Geometry check sheet. Reference: the model listing, model coordinates, mm. A direction names the side the tool comes from. Round coordinates to 2 decimals unless told otherwise and drop trailing zeros. Order: outer loops, then holes, each group sorted by start corner. A loop starts at its lowest first (then second) coordinate and runs counter-clockwise, first axis right, second up. Notation, with made-up numbers: (19.25, -22) - (76.25, -22) arc R25 cw to (76.25, -2) - close; hole circle Ø3 at (61.25, -19). An arc over 180 degrees is marked (long way). Return JSON: item names as keys, results as strings. Group by question number.
Q1. Draft check along Z on faces 1 (the flat face through (15, 11.847, 54)), 2 (the flat face through (-11, 36, 46.917)), 3 (the flat face through (-12, 22, 71.097)). Enter one of: pulls with the +Z half, pulls with the -Z half, needs draft (parallel to the pull), parting line crosses it, or undercut.
Q2. Sectioned sample at B-B, the plane y = 31.5. Record the cut outline in (x, z).
Q3. Sectioned sample at C-C, the plane y = 25.5. Record the cut outline in (x, z).
Q4. Tool access check on faces 4 (the flat face through (1, 22, 33.5)), 5 (the flat face through (-12, 22, 38.398)), 6 (the flat face through (4, 39.2, 93)), 7 (the flat face through (16.876, 37, 54)), 8 (the flat face through (1, 22, 58)). Record the directions out of +Z, -Z, +X, -X, +Y, -Y that give a thin tool (end or side, any length) a straight path to the whole face; none if there is none.
Q5. Gauge pin test, flat ends, axial feed: pin 1 Ø0.8 at (x, z) = (-12, 39.5) entering from -Y; pin 2 Ø3 at (y, z) = (2, 9) entering from -X; pin 3 Ø2.5 at (x, y) = (-10, 7.5) entering from -Z. Record the tip position at first contact, or that the pin passes through.
Q6. Material ranges on line 1 along Y through (x, z) = (12, 81.5); line 2 along Y through (x, z) = (5.5, 32); line 3 along Y through (x, z) = (-9.75, 55), recorded low to high.
Q7. Sectioned sample at D-D, the plane x = -8. Record the cut outline in (y, z).
```python
from build123d import *

# Parameters (mm, degrees)
BOSS_EXTRUDE1_DEPTH = 110
SKETCH2_W           = 33.5
SKETCH2_H           = 33.4
CUT_EXTRUDE1_DEPTH  = 10
SKETCH3_R           = 1.855174256
CUT_EXTRUDE3_DEPTH  = 10
SKETCH5_W           = 32.698767502
SKETCH5_H           = 33.097532959
BOSS_EXTRUDE2_DEPTH = 15
FILLET1_START       = 28.397979731
FILLET1_DEPTH       = 52.698767702
FILLET1_START_2     = -6.3183e-05
FILLET1_2_DEPTH     = 45.00011208
FILLET1_START_3     = 5.8
FILLET1_3_DEPTH     = 33.4
FILLET1_START_4     = 5.851542156
FILLET1_4_DEPTH     = 33.097532959
SKETCH6_R           = 13.931881445
CUT_EXTRUDE5_DEPTH  = 16
FILLET7_R           = 1
FILLET8_R           = 1
SKETCH8_W           = 6.973836054
SKETCH8_H           = 8.816669347
CUT_EXTRUDE6_DEPTH  = 9


with BuildPart() as part:
    # Sketch1 → Boss-Extrude1 (new body)
    with BuildSketch(Plane.XY):
        Polygon((0, 0), (0, 45), (20, 45), (20, 38.960548223), (16.876367343, 38.960548223), (16.876367343, 34.822386524), (20, 34.822386524), (20, 30.507676941), (10.5, 30.507676941), (10.5, 34.734112582), (13.516445061, 34.822386524), (13.516445061, 38.960548223), (10.5, 38.960548223), (4.092986166, 38.960548223), (4.092986166, 5.068373594), (10.5, 5.068373594), (13.538820233, 5.068373594), (13.538820233, 8.457591057), (10.5, 8.457591057), (10.5, 11.84680852), (20, 11.84680852), (20, 8.310671744), (16.876367343, 8.310671744), (16.876367343, 5.068373594), (20, 5.068373594), (20, 0), align=None)
    extrude(amount=BOSS_EXTRUDE1_DEPTH)

    # Sketch2 → Cut-Extrude1 (cut)
    with BuildSketch(Plane.ZY):
        with Locations((93.25, 22.5)):
            Rectangle(SKETCH2_W, SKETCH2_H)
        with Locations((16.75, 22.5)):
            Rectangle(SKETCH2_W, SKETCH2_H)
    extrude(amount=-CUT_EXTRUDE1_DEPTH, mode=Mode.SUBTRACT)

    # Sketch3 → Cut-Extrude3 (cut)
    with BuildSketch(Plane.ZY):
        with Locations((54.95102213, 22.327543377)):
            Circle(SKETCH3_R)
    extrude(amount=-CUT_EXTRUDE3_DEPTH, mode=Mode.SUBTRACT)

    # Sketch5 → Boss-Extrude2 (add)
    with BuildSketch(Plane.ZY):
        with Locations((54.747363582, 22.400308636)):
            Rectangle(SKETCH5_W, SKETCH5_H)
    extrude(amount=BOSS_EXTRUDE2_DEPTH)

    # Fillet1: read off the stored shape, not the designer's step
    # Fillet1 outline → Fillet1 (add)
    with BuildSketch(Plane.XY.offset(FILLET1_START)):
        with BuildLine():
            Line((0, 39.2), (2.35e-05, 45.000054671))
            ThreePointArc((2.35e-05, 45.000054671), (-3.686763576, 40.597721798), (-9.187208811, 38.949075115))
            Line((-9.187208811, 38.949075115), (0, 38.949075115))
            Line((0, 38.949075115), (0, 39.2))
        make_face()
        with BuildLine():
            Line((2.8807e-05, -6.3183e-05), (0, 5.851542156))
            Line((0, 5.851542156), (-9.098917382, 5.851542156))
            ThreePointArc((-9.098917382, 5.851542156), (-3.689848451, 4.262366926), (2.8807e-05, -6.3183e-05))
        make_face()
    extrude(amount=FILLET1_DEPTH)

    # Fillet1 2 outline → Fillet1 2 (cut)
    with BuildSketch(Plane(origin=(0, 0, 0), x_dir=(1, 0, 0), z_dir=(0, 1, 0)).offset(FILLET1_START_2)):
        with BuildLine():
            Line((-12, -28.397979731), (-12, -38.397979831))
            Line((-12, -38.397979831), (-10, -38.397979831))
            ThreePointArc((-10, -38.397979831), (-2.928932158, -35.469047613), (0, -28.397979745))
            Line((0, -28.397979745), (-12, -28.397979731))
        make_face()
        with BuildLine():
            Line((-10, -71.096747333), (-12, -71.096747333))
            Line((-12, -71.096747333), (-12, -81.096747433))
            Line((-12, -81.096747433), (0, -81.096747419))
            ThreePointArc((0, -81.096747419), (-2.928932158, -74.025679551), (-10, -71.096747333))
        make_face()
    extrude(amount=FILLET1_2_DEPTH, mode=Mode.SUBTRACT)

    # Fillet1 3 outline → Fillet1 3 (cut)
    with BuildSketch(Plane(origin=(0, 0, 0), x_dir=(1, 0, 0), z_dir=(0, 1, 0)).offset(FILLET1_START_3)):
        with BuildLine():
            Line((-1.399454076, -33.5), (0, -33.5))
            Line((0, -33.5), (0, -28.397979831))
            ThreePointArc((0, -28.397979831), (-0.356207716, -31.043215242), (-1.399454076, -33.5))
        make_face()
        with BuildLine():
            Line((0, -81.096747333), (0, -76.5))
            Line((0, -76.5), (-1.119126509, -76.5))
            ThreePointArc((-1.119126509, -76.5), (-0.283809005, -78.731238393), (0, -81.096747333))
        make_face()
    extrude(amount=FILLET1_3_DEPTH, mode=Mode.SUBTRACT)

    # Fillet1 4 outline → Fillet1 4 (add)
    with BuildSketch(Plane(origin=(0, 0, 0), x_dir=(1, 0, 0), z_dir=(0, 1, 0)).offset(FILLET1_START_4)):
        with BuildLine():
            Line((0, -38.397979831), (0, -33.5))
            Line((0, -33.5), (-1.399454076, -33.5))
            ThreePointArc((-1.399454076, -33.5), (-5.051272976, -37.087634649), (-10, -38.397979831))
            Line((-10, -38.397979831), (0, -38.397979831))
        make_face()
        with BuildLine():
            Line((-1.119126509, -76.5), (0, -76.5))
            Line((0, -76.5), (0, -71.096747333))
            Line((0, -71.096747333), (-10, -71.096747333))
            ThreePointArc((-10, -71.096747333), (-4.802282873, -72.55369538), (-1.119126509, -76.5))
        make_face()
    extrude(amount=FILLET1_4_DEPTH)

    # Sketch6 → Cut-Extrude5 (cut)
    with BuildSketch(Plane.ZY.offset(15)):
        with Locations((55, 21.872686564)):
            Circle(SKETCH6_R)
    extrude(amount=-CUT_EXTRUDE5_DEPTH, mode=Mode.SUBTRACT)

    # Fillet7
    fillet7_edges = [part.edges().sort_by_distance(p)[0] for p in [
        (20, 34.822386524, 55),
        (10.5, 34.734112582, 55),
    ]]
    fillet(fillet7_edges, radius=FILLET7_R)

    # Fillet8
    fillet8_edges = [part.edges().sort_by_distance(p)[0] for p in [
        (10.5, 8.457591057, 55),
        (20, 8.310671744, 55),
    ]]
    fillet(fillet8_edges, radius=FILLET8_R)

    # Sketch8 → Cut-Extrude6 (cut)
    with BuildSketch(Plane.ZY.offset(15)):
        with Locations((66.064245808, 34.540740441)):
            Rectangle(SKETCH8_W, SKETCH8_H)
        with Locations((43.430481356, 34.540740441)):
            Rectangle(SKETCH8_W, SKETCH8_H)
        with Locations((66.064245808, 10.25987683)):
            Rectangle(SKETCH8_W, SKETCH8_H)
        with Locations((43.430481356, 10.25987683)):
            Rectangle(SKETCH8_W, SKETCH8_H)
    extrude(amount=-CUT_EXTRUDE6_DEPTH, mode=Mode.SUBTRACT)


solid = part.part
```
Reply:
{
 "1": {"face 1": "needs draft", "face 2": "undercut", "face 3": "pulls with the +Z half"},
 "2": {"outline": "(-15, 38.4) - (-10, 38.4) arc R10 cw to (-1.4, 33.5) - (4.09, 33.5) - (4.09, 76.5) - (-1.12, 76.5) arc R10 cw to (-10, 71.1) - (-15, 71.1) - (-15, 69.55) - (-6, 69.55) - (-6, 65.07) - (1, 65.07) - (1, 44.93) - (-6, 44.93) - (-6, 39.94) - (-15, 39.94) - close; (10.5, 0) - (20, 0) - (20, 110) - (10.5, 110) - close"},
 "3": {"outline": "(-15, 38.4) - (-10, 38.4) arc R10 cw to (-1.4, 33.5) - (4.09, 33.5) - (4.09, 76.5) - (-1.12, 76.5) arc R10 cw to (-10, 71.1) - (-15, 71.1) - (-15, 68.45) - (1, 68.45) - (1, 41.55) - (-15, 41.55) - close"},
 "4": {"face 4": "-Z, -X", "face 5": "-Z, -X, +Y, -Y", "face 6": "+Z, -X", "face 7": "+Z, -Z, +X", "face 8": "-X"},
 "5": {"pin 1": "y = 5.85", "pin 2": "x = 0", "pin 3": "z = 38.32"},
 "6": {"line 1": "0 to 5.07, 8.46 to 11.85, 30.51 to 34.78, 38.96 to 45", "line 2": "0 to 5.07, 39.2 to 45", "line 3": "5.85 to 7.94, 35.8 to 38.95"},
 "7": {"outline": "(5.79, 38.2) - (39.02, 38.2) - (39.02, 71.3) - (5.79, 71.3) - close; hole (5.85, 39.94) - (14.67, 39.94) - (14.67, 43.08) arc R13.93 ccw to (30.13, 43.78) - (30.13, 39.94) - (38.95, 39.94) - (38.95, 46.92) - (33.22, 46.92) arc R13.93 ccw to (33.56, 62.58) - (38.95, 62.58) - (38.95, 69.55) - (30.13, 69.55) - (30.13, 66.22) arc R13.93 ccw to (14.67, 66.92) - (14.67, 69.55) - (5.85, 69.55) - (5.85, 62.58) - (10.18, 62.58) arc R13.93 ccw to (10.53, 46.92) - (5.85, 46.92) - close"}
}
